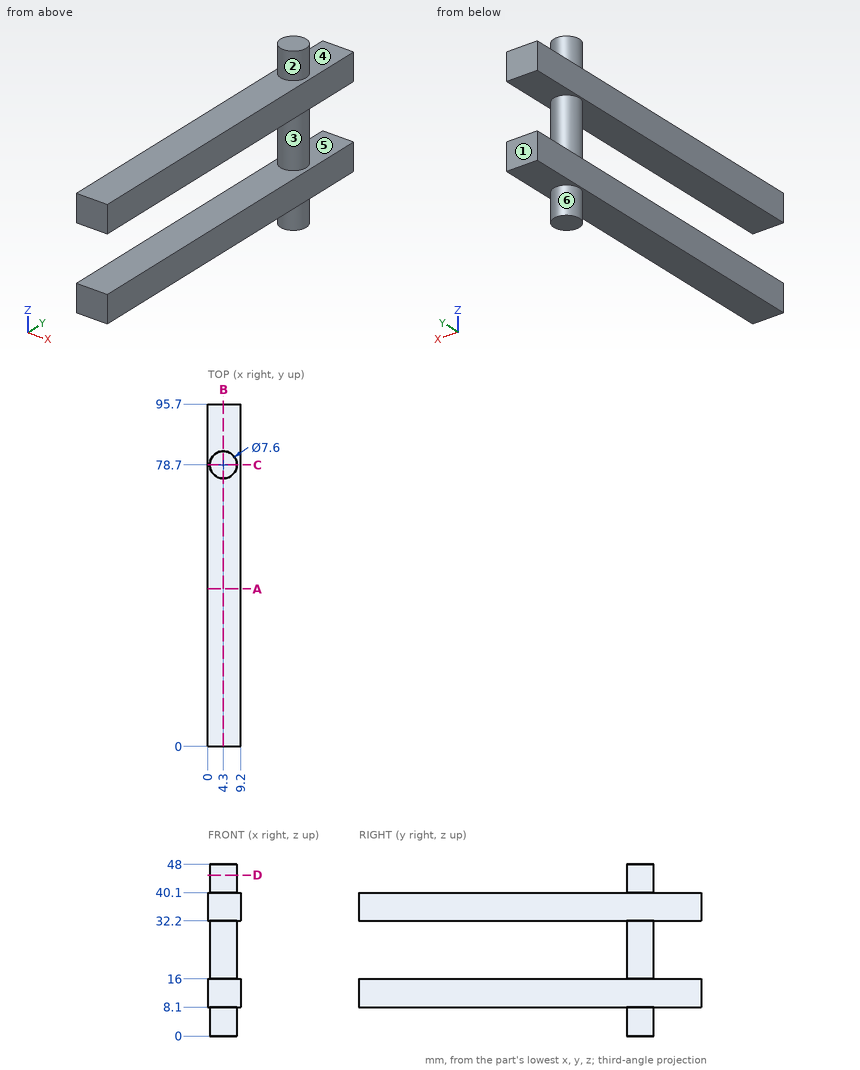
For this review, use the dimensioned drawing (mm, ordinates from the lowest corner) and the shaded views. A direction names the side the tool comes from. Give positions to 0.01 mm unless a question says otherwise; leave off trailing zeros. Loops run counter-clockwise (first coordinate to the right, second up) from the corner with the lowest first, then second, coordinate; pieces in that order, holes last.
Item 1: Insertion check: pin 1 (3 mm diameter, centred on x = 6.5, y = 59.5, fed in from +Z); pin 2 (3 mm diameter, centred on x = 3.5, z = 20.5, fed in from +Y); pin 3 (5 mm diameter, centred on x = 6.5, z = 27.5, fed in from -Y). Each pin has a flat end and moves straight along its axis. Give the tip position at first contact, or say it passes through.
Item 2: Take a section at D-D, the plane z = 45. State the section outline as (x, y) points, and give its area (3 significant figures).
Item 3: Take a section at B-B, the plane x = 4.3. State the section outline as (y, z) points.
Item 4: Draft analysis for pull direction Z (two halves, no side actions). For the marked faces 4, 5 and 6, state which applies: +Z half, -Z half, draft (parallel to the pull), parting line (faces both ways), or undercut.
Item 5: Tool access review of the marked faces 1, 2 and 3: name each direction out of +Z, -Z, +X, -X, +Y, -Y from which nothing blocks a thin tool from reaching the whole face with its end or side.
Item 6: For line 1 along Z through (x, y) = (7, 54.5); line 2 along Y through (x, z) = (2.75, 3.5); line 3 along Y through (x, z) = (2, 4), list the stretches that pass through material, from the lowest coordinate up.
Item 7: Take a section at C-C, the plane y = 78.7. State the section outline as (x, z) points.
Item 8: Take a section at A-A, the plane y = 44. State the section outline as (x, z) points.
Calculated:
1. pin 1: stops at z = 40.1
1. pin 2: stops at y = 82.5
1. pin 3: stops at y = 74.9
2. outline: circle Ø7.6 at (4.3, 78.7)
2. area: 45.4 mm2
3. outline: (0, 8.1) - (74.9, 8.1) - (74.9, 0) - (82.5, 0) - (82.5, 8.1) - (95.7, 8.1) - (95.7, 16) - (82.5, 16) - (82.5, 32.2) - (95.7, 32.2) - (95.7, 40.1) - (82.5, 40.1) - (82.5, 48) - (74.9, 48) - (74.9, 40.1) - (0, 40.1) - (0, 32.2) - (74.9, 32.2) - (74.9, 16) - (0, 16) - close
4. face 4: +Z half
4. face 5: undercut
4. face 6: draft
5. face 1: +Z, -Z, +X, -X, +Y
5. face 2: +Z
5. face 3: none
6. line 1: z = 8.1 to 16, 32.2 to 40.1
6. line 2: y = 75.23 to 82.17
6. line 3: y = 75.68 to 81.72
7. outline: (0, 8.1) - (0.5, 8.1) - (0.5, 0) - (8.1, 0) - (8.1, 8.1) - (9.2, 8.1) - (9.2, 16) - (8.1, 16) - (8.1, 32.2) - (9.2, 32.2) - (9.2, 40.1) - (8.1, 40.1) - (8.1, 48) - (0.5, 48) - (0.5, 40.1) - (0, 40.1) - (0, 32.2) - (0.5, 32.2) - (0.5, 16) - (0, 16) - close
8. outline: (0, 8.1) - (9.2, 8.1) - (9.2, 16) - (0, 16) - close; (0, 32.2) - (9.2, 32.2) - (9.2, 40.1) - (0, 40.1) - close
